Model file for the job. Use its own axes, mm. A direction names the side the tool comes from. Give positions to 0.01 mm unless a question says otherwise; leave off trailing zeros. Write each loop counter-clockwise with the first axis right and the second up, starting at its lowest first coordinate (ties: lowest second). Pieces come first, ordered by that corner, then holes. Notation, with made-up numbers: (5.25, 37.25) - (59.25, 37.25) arc R16 cw to (59.25, 47.25) - close; hole circle Ø7 at (-2, -4). An arc over 180 degrees is marked (long way). One line per item, written item: value. Start each with the question number.
(1) Cut at A-A, the plane y = 0. List the corners of the cut face in (x, z) (3 decimals).
(2) Cut at D-D, the plane z = -8.5. List the corners of the cut face in (x, y), and give its area (3 significant figures).
(3) Probe L1, parallel to Y at x = 3.75, z = 0 (3 decimals); L2, parallel to Y at x = 13.15, z = 0; L3, parallel to X at y = -10.5, z = 22. List the from-to ranges inside material, lowest first.
(4) Cut at B-B, the plane z = 0. List the corners of the cut face in (x, y) (3 decimals), and give its area (3 significant figures).
(5) Drop flat-ended pins along their axis: P1, Ø3, axis at y = -14.5, z = 14.5, coming from the -X side; P2, Ø8, axis at x = 7.5, z = 0, coming from the +Y side; P3, Ø13, axis at y = 0, z = 3, coming from the -X side; P4, Ø6, axis at x = 12, y = -14, coming from the +Z side. Give the stop position or say it passes through.
(6) Mould opens along Y. For faces 1 (the face through (2, -22.5, -0.1)), 2 (the face through (2, 22.5, 0.1)), 3 (the face through (1.26, -13.35, 13.24)) say: pulls with the +Y half, pulls with the -Y half, needs draft (parallel to the pull), parting line crosses it, or undercut.
(7) Cut at C-C, the plane x = 10.25. List the corners of the cut face in (y, z) (3 decimals), and give its area (3 significant figures).
(8) 3-axis set-ups, long thin cutter, end or side, ignore diameter. For faces 4 (the face through (11.5, -3, -3)), 5 (the face through (4, 17, 0)), 6 (the face through (1.26, 13.24, 13.35)): which of +Z, -Z, +X, -X, +Y, -Y reach the whole face in a straight line?
from build123d import *

# Parameters (mm, degrees)
SKETCH1_R                                       = 25
BOSS_EXTRUDE1_DEPTH                             = 4
SKETCH2_R                                       = 16.5
BOSS_EXTRUDE2_DEPTH                             = 10
SKETCH3_R                                       = 12.5
CUT_EXTRUDE1_DEPTH                              = 11.5
SKETCH4_R                                       = 4
CUT_EXTRUDE2_DEPTH                              = 4
M3_CLEARANCE_HOLE1_D                            = 3.4
M3_CLEARANCE_HOLE1_DEPTH                        = 10
CSK_FOR_M3_FLAT_HEAD_MACHINE_SCREW1_D           = 3.4
CSK_FOR_M3_FLAT_HEAD_MACHINE_SCREW1_CSINK_D     = 6.3
CSK_FOR_M3_FLAT_HEAD_MACHINE_SCREW1_CSINK_ANGLE = 90
CIRPATTERN1_COUNT                               = 4
SKETCH10_R                                      = 13.125
CUT_EXTRUDE3_DEPTH                              = 11.5
SKETCH12_R                                      = 4
CUT_EXTRUDE4_DEPTH                              = 10
FILLET1_R                                       = 1


with BuildPart() as part:
    # Sketch1 → Boss-Extrude1 (new body)
    with BuildSketch(Plane(origin=(0, 0, 0), x_dir=(0, 0, -1), z_dir=(1, 0, 0))):
        Circle(SKETCH1_R)
    extrude(amount=BOSS_EXTRUDE1_DEPTH)

    # Sketch2 → Boss-Extrude2 (add)
    with BuildSketch(Plane(origin=(4, 0, 0), x_dir=(0, 0, -1), z_dir=(1, 0, 0))):
        Circle(SKETCH2_R)
    extrude(amount=BOSS_EXTRUDE2_DEPTH)

    # Sketch3 → Cut-Extrude1 (cut)
    with BuildSketch(Plane.ZY):
        Circle(SKETCH3_R)
    extrude(amount=-CUT_EXTRUDE1_DEPTH, mode=Mode.SUBTRACT)

    # Sketch4 → Cut-Extrude2 (cut)
    with BuildSketch(Plane(origin=(14, 0, 0), x_dir=(0, 0, -1), z_dir=(1, 0, 0))):
        Circle(SKETCH4_R)
    extrude(amount=-CUT_EXTRUDE2_DEPTH, mode=Mode.SUBTRACT)

    # M3 Clearance Hole1
    with Locations(Plane(origin=(14, 0, 0), x_dir=(0, 0, -1), z_dir=(1, 0, 0))):
        with Locations((8.5, 0), (-8.5, 0)):
            Hole(M3_CLEARANCE_HOLE1_D / 2, depth=M3_CLEARANCE_HOLE1_DEPTH)

    # CSK for M3 Flat Head Machine Screw1 (through all)
    with Locations(Plane(origin=(4, 0, 0), x_dir=(0, 0, -1), z_dir=(1, 0, 0))):
        with Locations((-14.495689014, -14.495689014)):
            csk_for_m3_flat_head_machine_screw1 = CounterSinkHole(CSK_FOR_M3_FLAT_HEAD_MACHINE_SCREW1_D / 2, CSK_FOR_M3_FLAT_HEAD_MACHINE_SCREW1_CSINK_D / 2, counter_sink_angle=CSK_FOR_M3_FLAT_HEAD_MACHINE_SCREW1_CSINK_ANGLE)

    # CirPattern1: CSK for M3 Flat Head Machine Screw1 ×4 about axis
    cirpattern1_axis = Axis((0, 0, 0), (1, 0, 0))
    for i in range(1, CIRPATTERN1_COUNT):
        add(csk_for_m3_flat_head_machine_screw1.rotate(cirpattern1_axis, i * 360 / CIRPATTERN1_COUNT), mode=Mode.SUBTRACT)

    # Sketch10 → Cut-Extrude3 (cut)
    with BuildSketch(Plane.ZY):
        Circle(SKETCH10_R)
    extrude(amount=-CUT_EXTRUDE3_DEPTH, mode=Mode.SUBTRACT)

    # Sketch12 → Cut-Extrude4 (cut)
    with BuildSketch(Plane(origin=(4, 0, 0), x_dir=(0, 0, -1), z_dir=(1, 0, 0))):
        with Locations((0, 26.5)):
            Circle(SKETCH12_R)
        with Locations((0, -26.5)):
            Circle(SKETCH12_R)
    extrude(amount=-CUT_EXTRUDE4_DEPTH, mode=Mode.SUBTRACT)

    # Fillet1
    fillet1_edges = [part.edges().sort_by_distance(p)[0] for p in [
        (2, 24.740566038, -3.592268383),
        (2, 24.740566038, 3.592268383),
        (2, -24.740566038, 3.592268383),
        (2, -24.740566038, -3.592268383),
    ]]
    fillet(fillet1_edges, radius=FILLET1_R)


solid = part.part
Answers follow:
1. outline: (0, -25) - (4, -25) - (4, -16.5) - (14, -16.5) - (14, -10.2) - (11.5, -10.2) - (11.5, -13.125) - (0, -13.125) - close; (0, 13.125) - (11.5, 13.125) - (11.5, 10.2) - (14, 10.2) - (14, 16.5) - (4, 16.5) - (4, 25) - (0, 25) - close; (11.5, -6.8) - (14, -6.8) - (14, -4) - (11.5, -4) - close; (11.5, 4) - (14, 4) - (14, 6.8) - (11.5, 6.8) - close
2. outline: (0, -23.51) - (4, -23.51) - (4, -14.14) - (14, -14.14) - (14, -1.7) - (11.5, -1.7) - (11.5, -10) - (0, -10) - close; (0, 10) - (11.5, 10) - (11.5, 1.7) - (14, 1.7) - (14, 14.14) - (4, 14.14) - (4, 23.51) - (0, 23.51) - close
2. area: 232 mm²
3. L1: y = -22.5 to -13.125, 13.125 to 22.5
3. L2: y = -16.5 to -4, 4 to 16.5
3. L3: x = 0 to 4
4. outline: (0, -22.5) - (4, -22.5) - (4, -16.5) - (14, -16.5) - (14, -4) - (11.5, -4) - (11.5, -13.125) - (0, -13.125) - close; (0, 13.125) - (11.5, 13.125) - (11.5, 4) - (14, 4) - (14, 16.5) - (4, 16.5) - (4, 22.5) - (0, 22.5) - close
4. area: 188 mm²
5. P1: passes through
5. P2: stops at y = 23
5. P3: stops at x = 11.5
5. P4: stops at z = 12.3
6. face 1: pulls with the -Y half
6. face 2: pulls with the +Y half
6. face 3: undercut
7. outline: circle Ø33 at (0, 0); hole circle Ø26.25 at (0, 0)
7. area: 314 mm²
8. face 4: -X
8. face 5: +X
8. face 6: +X, -X
